from build123d import *

# Parameters (mm, degrees)
F0_W     = 6
F0_H     = 15
F0_W_2   = 36
F1_DEPTH = 4
F2_DEPTH = 25
F4_DEPTH = 15
F5_W     = 36
F5_H     = 3
F6_DEPTH = 20
F7_R     = 2
F8_DEPTH = 3


with BuildPart() as f1:
    # F0 (on Top) → F1 (new body)
    with BuildSketch(Plane.XY):
        with Locations((-21, -7.5)):
            Rectangle(F0_W, F0_H)
        with Locations((0, -7.5)):
            Rectangle(F0_W_2, F0_H)
        with Locations((21, -7.5)):
            Rectangle(F0_W, F0_H)
    extrude(amount=-F1_DEPTH)

    # F0 (on Top) → F2 (join)
    with BuildSketch(Plane.XY):
        with Locations((-21, -7.5)):
            Rectangle(F0_W, F0_H)
        with Locations((21, -7.5)):
            Rectangle(F0_W, F0_H)
    extrude(amount=-F2_DEPTH)

    # F3 (on face) → F4 (join, through all)
    with BuildSketch(Plane.XZ.offset(15)):
        Polygon((24, -29), (24, -25), (18, -25), (14, -25), (14, -27), align=None)
        Polygon((-18, -25), (-24, -25), (-24, -29), (-14, -27), (-14, -25), align=None)
    extrude(amount=-F4_DEPTH)

    # F5 (on Top) → F6 (join)
    with BuildSketch(Plane.XY):
        with Locations((0, -1.5)):
            Rectangle(F5_W, F5_H)
    extrude(amount=F6_DEPTH)

    # F7 (on face) → F8 (cut, through all)
    with BuildSketch(Plane(origin=(0, 0, 0), x_dir=(-1, 0, 0), z_dir=(0, 1, 0))):
        with Locations((0, 15)):
            Circle(F7_R)
    extrude(amount=-F8_DEPTH, mode=Mode.SUBTRACT)


solid = f1.part
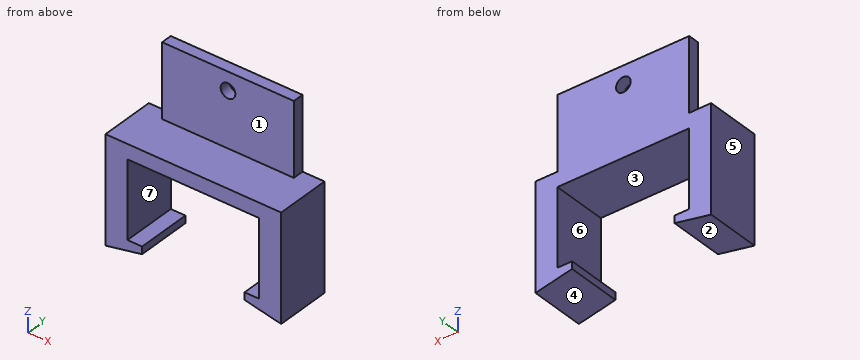
Geometry: final body of the model. Coordinates: model frame, mm. Face numbers are marked on the shaded views. A direction names the side the tool comes from. Give positions to 0.01 mm unless a question says otherwise; leave off trailing zeros. Order: outer loops, then holes, each group sorted by start corner. A loop starts at its lowest first (then second) coordinate and runs counter-clockwise, first axis right, second up. Notation, with made-up numbers: (59, -2) - (110, -2) arc R23 cw to (110, 17) - close; hole circle Ø7 at (60, -26.5). An arc over 180 degrees is marked (long way). Use CSV: the item, a comma, the result in double quotes.
1. Section query B-B (x = 0). Output: boundary loops of the cut face in (y, z), plus the area to 3 significant figures.
Answers below:
outline,"(-15, -4) - (0, -4) - (0, 13) - (-3, 13) - (-3, 0) - (-15, 0) - close; (-3, 17) - (0, 17) - (0, 20) - (-3, 20) - close"
area,"108 mm2"
2. Mould query, pull axis Z, two halves, no side actions, for the marked faces 4, 5, 6 and 7. Classes: +Z half, -Z half, draft (parallel to the pull), parting line (faces both ways), or undercut.
Answers below:
face 4,"-Z half"
face 5,"draft"
face 6,"undercut"
face 7,"undercut"
3. Section query C-C (y = -1). Output: boundary loops of the cut face in (x, z), plus the area to 3 significant figures.
Answers below:
outline,"(-24, -29) - (-14, -27) - (-14, -25) - (-18, -25) - (-18, -4) - (18, -4) - (18, -25) - (14, -25) - (14, -27) - (24, -29) - (24, 0) - (18, 0) - (18, 20) - (-18, 20) - (-18, 0) - (-24, 0) - close; hole circle Ø4 at (0, 15)"
area,"1,210 mm2"
4. Section query A-A (z = 15). Output: boundary loops of the cut face in (x, y).
Answers below:
outline,"(-18, -3) - (-2, -3) - (-2, 0) - (-18, 0) - close; (2, -3) - (18, -3) - (18, 0) - (2, 0) - close"
5. Access query for the marked faces 1, 2 and 3. Directions: +Z, -Z, +X, -X, +Y, -Y. A direction counts if a zero-diameter tool reaches every point of the face in a straight line with its end or side. Return the directions, or none.
Answers below:
face 1,"+Z, +X, -X, -Y"
face 2,"-Z, +Y, -Y"
face 3,"+Y, -Y"
6. Contact query for flat-ended pins moving along their axis: pin 1 (4.5 mm diameter, centred on x = -2, y = -8, fed in from -Z); pin 2 (3.5 mm diameter, centred on y = -1, z = 9.5, fed in from +X); pin 3 (2 mm diameter, centred on x = -16.5, y = -7, fed in from +Z). Output: stop coordinate, or through.
Answers below:
pin 1,"z = -4"
pin 2,"x = 18"
pin 3,"z = 0"
7. Section query D-D (z = -10). Output: boundary loops of the cut face in (x, y).
Answers below:
outline,"(-24, -15) - (-18, -15) - (-18, 0) - (-24, 0) - close; (18, -15) - (24, -15) - (24, 0) - (18, 0) - close"
8. Material intervals for line 1 along Z through (x, y) = (0, -1.1); line 2 along X through (y, z) = (-4.75, -8); line 3 along Y through (x, z) = (-16, 2), sorted ascending. Write a range as from..to.
Answers below:
line 1,"-4..13, 17..20"
line 2,"-24..-18, 18..24"
line 3,"-3..0"
